Input: part model. Units: mm. Frame: model coordinates. A direction names the side the tool comes from. Give positions to 0.01 mm unless a question says otherwise; leave off trailing zeros. Write each loop counter-clockwise with the first axis right and the second up, starting at its lowest first coordinate (ties: lowest second). Pieces come first, ordered by that corner, then holes.
```python
from build123d import *

# Parameters (mm, degrees)
VYSUNOUT_TENKOST_NN_1_DEPTH       = 180
SKICA5_W                          = 60
SKICA5_H                          = 1
P_IDAT_VYSUNUT_M3_DEPTH           = 180
SKICA6_W                          = 40
SKICA6_H                          = 30
ODEBRAT_VYSUNUT_M2_DEPTH          = 3
SKICA7_W                          = 6
SKICA7_H                          = 6
P_IDAT_VYSUNUT_M4_DEPTH           = 5
SKICA8_R                          = 1.4
ODEBRAT_VYSUNUT_M3_DEPTH          = 5
SKICA9_R                          = 5.25
ODEBRAT_VYSUNUT_M4_DEPTH          = 225.510578815
P_IDAT_VYSUNUT_M7_DEPTH           = 6
SKICA16_R                         = 1.4
ODEBRAT_VYSUNUT_M13_DEPTH         = 10
P_IDAT_VYSUNUT_M8_DEPTH           = 6
SKICA18_R                         = 1.4
ODEBRAT_VYSUNUT_M14_DEPTH         = 16
P_IDAT_VYSUNUT_M9_DEPTH           = 6
SKICA20_R                         = 1.4
ODEBRAT_VYSUNUT_M15_DEPTH         = 16
ODEBRAT_START                     = -25
ODEBRAT_VYSUNUT_M16_DEPTH         = 8
P_IDAT_VYSUNUT_M10_DEPTH          = 30
SKICA23_R                         = 5.25
ODEBRAT_VYSUNUT_M17_DEPTH         = 224.705721876
D_RY_PRO_KOL_K_VELIKOST_MM1_D     = 3
D_RY_PRO_KOL_K_VELIKOST_MM1_DEPTH = 10
D_RY_PRO_KOL_K_VELIKOST_MM1_TIP   = 0.901290929
SKICA29_W                         = 6
SKICA29_H                         = 3
ODEBRAT_VYSUNUT_M18_DEPTH         = 10
SKICA30_W                         = 24
SKICA30_H                         = 15
ODEBRAT_VYSUNUT_M19_DEPTH         = 5


with BuildPart() as part:
    # Skica4 → Vysunout tenkostěnný1 (new body)
    with BuildSketch(Plane(origin=(0, 0, 0), x_dir=(0, 0, -1), z_dir=(1, 0, 0))):
        Polygon((0, 0), (30, 0), (30, 28), (59, 28), (59, 58), (60.5, 58), (60.5, 26.5), (31.5, 26.5), (31.5, -1.5), (0, -1.5), align=None)
    vysunout_tenkost_nn_1 = extrude(amount=VYSUNOUT_TENKOST_NN_1_DEPTH)

    # Zrcadlit1: Vysunout tenkostěnný1 across plane
    add(vysunout_tenkost_nn_1.mirror(Plane(origin=(180, -1.5, 0), x_dir=(1, 0, 0), z_dir=(0, 0, 1))))

    # Skica5 → Přidat vysunutím3 (add)
    with BuildSketch(Plane.ZY):
        with Locations((0, 27.5)):
            Rectangle(SKICA5_W, SKICA5_H)
    extrude(amount=-P_IDAT_VYSUNUT_M3_DEPTH)

    # Skica6 → Odebrat vysunutím2 (cut)
    with BuildSketch(Plane(origin=(0, 28, 0), x_dir=(1, 0, 0), z_dir=(0, 1, 0))):
        with Locations((180, 0)):
            Rectangle(SKICA6_W, SKICA6_H)
    extrude(amount=-ODEBRAT_VYSUNUT_M2_DEPTH, mode=Mode.SUBTRACT)

    # Skica7 → Přidat vysunutím4 (add)
    with BuildSketch(Plane.ZY):
        with Locations((-56, 31)):
            Rectangle(SKICA7_W, SKICA7_H)
        with Locations((-56, 55)):
            Rectangle(SKICA7_W, SKICA7_H)
        with Locations((56, 55)):
            Rectangle(SKICA7_W, SKICA7_H)
        with Locations((56, 31)):
            Rectangle(SKICA7_W, SKICA7_H)
        with Locations((27, 3)):
            Rectangle(SKICA7_W, SKICA7_H)
        with Locations((-27, 3)):
            Rectangle(SKICA7_W, SKICA7_H)
    extrude(amount=-P_IDAT_VYSUNUT_M4_DEPTH)

    # Skica8 → Odebrat vysunutím3 (cut)
    with BuildSketch(Plane.ZY):
        with Locations((-56, 55)):
            Circle(SKICA8_R)
        with Locations((-56, 31)):
            Circle(SKICA8_R)
        with Locations((-27, 3)):
            Circle(SKICA8_R)
        with Locations((27, 3)):
            Circle(SKICA8_R)
        with Locations((56, 31)):
            Circle(SKICA8_R)
        with Locations((56, 55)):
            Circle(SKICA8_R)
    extrude(amount=-ODEBRAT_VYSUNUT_M3_DEPTH, mode=Mode.SUBTRACT)

    # Skica9 → Odebrat vysunutím4 (cut, through all)
    with BuildSketch(Plane(origin=(0, 0, -60.5), x_dir=(-1, 0, 0), z_dir=(0, 0, -1))):
        with Locations((-135, 45.5)):
            Circle(SKICA9_R)
    extrude(amount=-ODEBRAT_VYSUNUT_M4_DEPTH, mode=Mode.SUBTRACT)

    # Skica15 → Přidat vysunutím7 (add)
    with BuildSketch(Plane.XY.offset(-30)):
        Polygon((180, 0), (180, 6), (177, 6), (169.849478444, 0), align=None)
    p_idat_vysunut_m7 = extrude(amount=P_IDAT_VYSUNUT_M7_DEPTH)

    # Skica16 → Odebrat vysunutím13 (cut)
    with BuildSketch(Plane(origin=(180, 0, 0), x_dir=(0, 0, -1), z_dir=(1, 0, 0))):
        with Locations(Location((27, 3, 0), (0, 0, 180))):
            Circle(SKICA16_R)
    odebrat_vysunut_m13 = extrude(amount=-ODEBRAT_VYSUNUT_M13_DEPTH, mode=Mode.SUBTRACT)

    # Skica17 → Přidat vysunutím8 (add)
    with BuildSketch(Plane.XY.offset(-59)):
        Polygon((180, 28), (180, 34), (177, 34), (169.849478444, 28), align=None)
    p_idat_vysunut_m8 = extrude(amount=P_IDAT_VYSUNUT_M8_DEPTH)

    # Skica18 → Odebrat vysunutím14 (cut)
    with BuildSketch(Plane(origin=(180, 0, 0), x_dir=(0, 0, -1), z_dir=(1, 0, 0))):
        with Locations(Location((56, 31, 0), (0, 0, 180))):
            Circle(SKICA18_R)
    odebrat_vysunut_m14 = extrude(amount=-ODEBRAT_VYSUNUT_M14_DEPTH, mode=Mode.SUBTRACT)

    # Skica19 → Přidat vysunutím9 (add)
    with BuildSketch(Plane(origin=(0, 58, 0), x_dir=(1, 0, 0), z_dir=(0, 1, 0))):
        Polygon((180, 59), (177, 59), (169.849478444, 59), (177, 53), (180, 53), align=None)
    p_idat_vysunut_m9 = extrude(amount=-P_IDAT_VYSUNUT_M9_DEPTH)

    # Skica20 → Odebrat vysunutím15 (cut)
    with BuildSketch(Plane(origin=(180, 0, 0), x_dir=(0, 0, -1), z_dir=(1, 0, 0))):
        with Locations(Location((56, 55, 0), (0, 0, 180))):
            Circle(SKICA20_R)
    odebrat_vysunut_m15 = extrude(amount=-ODEBRAT_VYSUNUT_M15_DEPTH, mode=Mode.SUBTRACT)

    # Zrcadlit2: Přidat vysunutím7, Odebrat vysunutím13, Přidat vysunutím8, Odebrat vysunutím14, Přidat vysunutím9, Odebrat vysunutím15 across plane
    add(p_idat_vysunut_m7.mirror(Plane.XY))
    add(odebrat_vysunut_m13.mirror(Plane.XY), mode=Mode.SUBTRACT)
    add(p_idat_vysunut_m8.mirror(Plane.XY))
    add(odebrat_vysunut_m14.mirror(Plane.XY), mode=Mode.SUBTRACT)
    add(p_idat_vysunut_m9.mirror(Plane.XY))
    add(odebrat_vysunut_m15.mirror(Plane.XY), mode=Mode.SUBTRACT)

    # Skica21 → Odebrat vysunutím16 (cut)
    with BuildSketch(Plane.XZ.offset(1.5).offset(ODEBRAT_START)):
        Polygon((62, -15), (52, -25), (50, -25), (50, 25), (52, 25), (62, 15), align=None)
        Polygon((86, -25), (84, -25), (84, 25), (86, 25), (96, 15), (96, -15), align=None)
    extrude(amount=-ODEBRAT_VYSUNUT_M16_DEPTH, mode=Mode.SUBTRACT)

    # Skica22 → Přidat vysunutím10 (add)
    with BuildSketch(Plane(origin=(0, 28, 0), x_dir=(1, 0, 0), z_dir=(0, 1, 0))):
        Polygon((117.053847577, 59), (150.25, 59), (150.25, 56), (122.25, 56), align=None)
        Polygon((122.25, -56), (117.053847577, -59), (150.25, -59), (150.25, -56), align=None)
    extrude(amount=P_IDAT_VYSUNUT_M10_DEPTH)

    # Skica23 → Odebrat vysunutím17 (cut, through all)
    with BuildSketch(Plane.XY.offset(59)):
        with Locations(Location((135, 45.5, 0), (0, 0, 180))):
            Circle(SKICA23_R)
    extrude(amount=-ODEBRAT_VYSUNUT_M17_DEPTH, mode=Mode.SUBTRACT)

    # Díry pro kolík, velikost mm1
    with Locations(Plane(origin=(0, 28, 0), x_dir=(1, 0, 0), z_dir=(0, 1, 0))):
        with Locations((155, -37.5), (115, -37.5), (115, 37.5), (155, 37.5)):
            Hole(D_RY_PRO_KOL_K_VELIKOST_MM1_D / 2, depth=D_RY_PRO_KOL_K_VELIKOST_MM1_DEPTH)
            with Locations((0, 0, -(D_RY_PRO_KOL_K_VELIKOST_MM1_DEPTH + D_RY_PRO_KOL_K_VELIKOST_MM1_TIP / 2))):  # 118° drill point
                Cone(0, D_RY_PRO_KOL_K_VELIKOST_MM1_D / 2, D_RY_PRO_KOL_K_VELIKOST_MM1_TIP, mode=Mode.SUBTRACT)

    # Skica29 → Odebrat vysunutím18 (cut)
    with BuildSketch(Plane.XY.offset(31.5)):
        with Locations((23, 10)):
            Rectangle(SKICA29_W, SKICA29_H)
    extrude(amount=-ODEBRAT_VYSUNUT_M18_DEPTH, mode=Mode.SUBTRACT)

    # Skica30 → Odebrat vysunutím19 (cut)
    with BuildSketch(Plane.XY.offset(60.5)):
        with Locations((47, 41.5)):
            Rectangle(SKICA30_W, SKICA30_H)
    extrude(amount=-ODEBRAT_VYSUNUT_M19_DEPTH, mode=Mode.SUBTRACT)


solid = part.part
```
Q1. Material intervals for line 1 along X through (y, z) = (27.05, 37.5); line 2 along Y through (x, z) = (2.85, -27); line 3 along Y through (x, z) = (144.5, 15.5), sorted ascending.
Q2. Section B-B, the plane y = 36.5. Return the cut outline in (x, z).
Q3. Section C-C, the plane x = 78. Return the cut outline in (y, z), then the cut area to 4 significant figures.
Q4. Pin query (flat end, axial travel): pin 1 (1.5 mm diameter, centred on x = 2, z = 28.5, fed in from +Y); pin 2 (1.5 mm diameter, centred on y = 35.5, z = -58, fed in from +X); pin 3 (2 mm diameter, centred on x = 106, y = 4.5, fed in from -Z); pin 4 (8 mm diameter, centred on y = 24.5, z = -30.5, fed in from -X). Return the tip coordinate at first contact, or that it passes through.
Q5. Section D-D, the plane y = 45.5. Return the cut outline in (x, z), then the cut area to 3 significant figures.
Q6. Mould query, pull axis Z, two halves, no side actions, for faces 5 (the flat face through (180, 24, -31)), 6 (the flat face through (69, 27, 0)). Classes: +Z half, -Z half, draft (parallel to the pull), parting line (faces both ways), or undercut.
Q7. Access query for faces 1 (the flat face through (140, 43, 56)), 2 (the flat face through (2, 55, 53)), 3 (the flat face through (2, 6, 27)), 4 (the flat face through (89, 13, 30)). Directions: +Z, -Z, +X, -X, +Y, -Y. A direction counts if a zero-diameter tool reaches every point of the face in a straight line with its end or side. Return the directions, or none.
Q8. Section A-A, the plane y = 18. Return the cut outline in (x, z), then the cut area to 3 significant figures.
Solutions:
1. line 1: x = 0 to 113.5, 116.5 to 153.5, 156.5 to 180
1. line 2: y = -1.5 to 1.6, 4.4 to 6, 27 to 28
1. line 3: y = -1.5 to 0, 27 to 28
2. outline: (0, -60.5) - (180, -60.5) - (180, -59) - (150.25, -59) - (150.25, -56) - (122.25, -56) - (117.05, -59) - (0, -59) - close; (0, 59) - (35, 59) - (35, 60.5) - (0, 60.5) - close; (59, 59) - (117.05, 59) - (122.25, 56) - (150.25, 56) - (150.25, 59) - (180, 59) - (180, 60.5) - (59, 60.5) - close
3. outline: (-1.5, -31.5) - (26.5, -31.5) - (26.5, -60.5) - (58, -60.5) - (58, -59) - (28, -59) - (28, 59) - (58, 59) - (58, 60.5) - (26.5, 60.5) - (26.5, 31.5) - (-1.5, 31.5) - close; hole (0, -30) - (27, -30) - (27, 30) - (0, 30) - close
3. area: 415.5 mm2
4. pin 1: stops at y = 28
4. pin 2: stops at x = 150.25
4. pin 3: stops at z = -31.5
4. pin 4: stops at x = 0
5. outline: (0, -60.5) - (129.75, -60.5) - (129.75, -56) - (122.25, -56) - (117.05, -59) - (0, -59) - close; (0, 59) - (35, 59) - (35, 60.5) - (0, 60.5) - close; (59, 59) - (117.05, 59) - (122.25, 56) - (129.75, 56) - (129.75, 60.5) - (59, 60.5) - close; (140.25, -60.5) - (180, -60.5) - (180, -59) - (150.25, -59) - (150.25, -56) - (140.25, -56) - close; (140.25, 56) - (150.25, 56) - (150.25, 59) - (180, 59) - (180, 60.5) - (140.25, 60.5) - close
5. area: 593 mm2
6. face 5: draft
6. face 6: undercut
7. face 1: +Y
7. face 2: +X, -X, +Y
7. face 3: +X, -X
7. face 4: none
8. outline: (0, -31.5) - (180, -31.5) - (180, -30) - (0, -30) - close; (0, 30) - (180, 30) - (180, 31.5) - (0, 31.5) - close
8. area: 540 mm2
